```python
from build123d import *

# Parameters (mm, degrees)
F0_W     = 600
F0_H     = 897
F1_DEPTH = 20
F2_W     = 600
F2_H     = 295
F2_H_2   = 480
F3_DEPTH = 20


with BuildPart() as f1:
    # F0 (on Front) → F1 (new body)
    with BuildSketch(Plane.XZ):
        Rectangle(F0_W, F0_H)
    extrude(amount=F1_DEPTH)

    # F2 (on face) → F3 (join)
    with BuildSketch(Plane.XZ.offset(20)):
        with Locations((0, 301)):
            Rectangle(F2_W, F2_H)
        with Locations((0, -119.5)):
            Rectangle(F2_W, F2_H_2)
    extrude(amount=F3_DEPTH)


solid = f1.part
```
Geometry: final body of the model. Coordinates: model frame, mm. A direction names the side the tool comes from. Round coordinates to 2 decimals unless told otherwise and drop trailing zeros. Loops run counter-clockwise (first coordinate to the right, second up) from the corner with the lowest first, then second, coordinate; pieces in that order, holes last. Notation, with made-up numbers: (3, -32) -> (37, -32) arc R15 cw to (37, -23) -> close; hole circle Ø10 at (-29, 81.5). An arc over 180 degrees is marked (long way). Write each question's results on one line, items separated by ' | '.
Item 1: Cut plane B-B on x = 192.5. Return the cut outline in (y, z).
Answers below:
outline: (-40, -359.5) -> (-20, -359.5) -> (-20, -448.5) -> (0, -448.5) -> (0, 448.5) -> (-40, 448.5) -> (-40, 153.5) -> (-20, 153.5) -> (-20, 120.5) -> (-40, 120.5) -> close
Item 2: Pull-direction query (Z, two-part tool) for faces 1 (the face through (-300, -20, -6)), 2 (the face through (-4, -20, 448.5)), 3 (the face through (-4, -30, 120.5)); classes: pulls with the +Z half, pulls with the -Z half, needs draft (parallel to the pull), parting line crosses it, or undercut.
Answers below:
face 1: needs draft | face 2: pulls with the +Z half | face 3: undercut
Item 3: Cut plane A-A on y = -31. Return the cut outline in (x, z).
Answers below:
outline: (-300, -359.5) -> (300, -359.5) -> (300, 120.5) -> (-300, 120.5) -> close; (-300, 153.5) -> (300, 153.5) -> (300, 448.5) -> (-300, 448.5) -> close
Item 4: Line query: probe 1 along Z at (x, y) = (-99, -24.5); probe 2 along Y at (x, z) = (147.5, 122). Output: solid intervals per line, ascending. Write a range as [from, to].
Answers below:
probe 1: z = [-359.5, 120.5], [153.5, 448.5] | probe 2: y = [-20, 0]
Item 5: Set-up query: faces 4 (the face through (-4, 0, 6)), 5 (the face through (-4, -20, 137)), 6 (the face through (-4, -20, -403)). Return all of +Z, -Z, +X, -X, +Y, -Y with unobstructed straight access to the full face (end or side cutting, diameter ignored); none if empty.
Answers below:
face 4: +Z, -Z, +X, -X, +Y | face 5: +X, -X, -Y | face 6: -Z, +X, -X, -Y
Item 6: Pin query (flat end, axial travel): pin 1 Ø2 at (x, y) = (-77.5, -23) entering from -Z. Return the tip coordinate at first contact, or that it passes through.
Answers below:
pin 1: stops at z = -359.5
